Source: CAD feature listing. Evaluate the final solid. Frame: model axes, mm. A direction names the side the tool comes from. Coordinates: 2 decimals unless noted, no trailing zeros. Write each loop counter-clockwise with the first axis right and the second up, starting at its lowest first coordinate (ties: lowest second). Pieces come first, ordered by that corner, then holes. Notation, with made-up numbers: M -23,4 L 5,4 A10 cw 5,9 Z; hole C -31.5,48.25 d7. An arc over 180 degrees is marked long. Answer as CSV lines item,"result". Start each with the question number.
1. Line query: probe 1 along Y at (x, z) = (12, 187.17); probe 2 along Z at (x, y) = (-11, 0); probe 3 along Z at (x, y) = (0, 0). Output: solid intervals per line, ascending. Write a range as [from, to].
2. Mould query, pull axis Y, two halves, no side actions, for faces 4 (the face through (0.993, 2.628, 178.824)), 5 (the face through (26, 0, 145)), 6 (the face through (-2.17, -9.76, -39.44)). Classes: pulls with the +Y half, pulls with the -Y half, needs draft (parallel to the pull), parting line crosses it, or undercut.
3. Contact query for flat-ended pins moving along their axis: pin 1 Ø4.5 at (y, z) = (21.5, 159.5) entering from -X; pin 2 Ø10.5 at (y, z) = (0, 187.17) entering from -X; pin 3 Ø1.5 at (x, y) = (-12.5, 1.5) entering from -Z; pin 4 Ø4.5 at (x, z) = (-24, 96.5) entering from +Y. Output: stop coordinate, or through.
4. Section B-B on x = 0. Return the cut outline in (y, z), plus the area to 3 significant figures.
5. Section A-A on z = 187.17. Return the cut outline in (x, y) (3 decimals), plus the area to 3 significant figures.
6. Section C-C on z = 271. Return the cut outline in (x, y).
7. Reachability of faces 1 (the face through (-22, 20, 145)), 2 (the face through (22, 20, 145)), 3 (the face through (0, 27.5, 145)) from +Z, -Z, +X, -X, +Y, -Y: full face, straight path, thin tool, end or side. Return the list, or none.
8. Section D-D on y = 24. Return the cut outline in (x, z), plus the area to 3 significant figures.
```python
from build123d import *

# Parameters (mm, degrees)
BOSS_EXTRUDE1_DEPTH          = 295
SKETCH3_R                    = 10
BOSS_EXTRUDE3_DEPTH          = 80
M20_TAPPED_HOLE1_D           = 17.5
M20_TAPPED_HOLE1_CSINK_D     = 20.05
M20_TAPPED_HOLE1_CSINK_ANGLE = 90


with BuildPart() as part:
    # Sketch1 → Boss-Extrude1 (new body)
    with BuildSketch(Plane.XY):
        Polygon((-26, -12.5), (26, -12.5), (26, 12.5), (22, 12.5), (22, 27.5), (-22, 27.5), (-22, 12.5), (-26, 12.5), align=None)
    extrude(amount=BOSS_EXTRUDE1_DEPTH)

    # Sketch3 → Boss-Extrude3 (add)
    with BuildSketch(Plane.XY):
        Circle(SKETCH3_R)
    extrude(amount=-BOSS_EXTRUDE3_DEPTH)

    # M20 Tapped Hole1 (through all)
    with Locations(Plane.ZY.offset(26)):
        with Locations((187.17, 0)):
            CounterSinkHole(M20_TAPPED_HOLE1_D / 2, M20_TAPPED_HOLE1_CSINK_D / 2, counter_sink_angle=M20_TAPPED_HOLE1_CSINK_ANGLE)


solid = part.part
```
Values:
1,probe 1,"[-12.5, -8.75], [8.75, 27.5]"
1,probe 2,"[0, 178.42], [195.92, 295]"
1,probe 3,"[-80, 178.42], [195.92, 295]"
2,face 4,"undercut"
2,face 5,"needs draft"
2,face 6,"parting line crosses it"
3,pin 1,"x = -22"
3,pin 2,"through"
3,pin 3,"z = 0"
3,pin 4,"y = 27.5"
4,outline,"M -12.5,0 L -10,0 L -10,-80 L 10,-80 L 10,0 L 27.5,0 L 27.5,295 L -12.5,295 Z; hole C 0,187.17 d17.5"
4,area,"13,200 mm²"
5,outline,"M -26,-12.5 L 26,-12.5 L 26,-8.75 L -24.725,-8.75 L -26,-10.025 Z; M -26,10.025 L -24.725,8.75 L 26,8.75 L 26,12.5 L 22,12.5 L 22,27.5 L -22,27.5 L -22,12.5 L -26,12.5 Z"
5,area,"1,050 mm²"
6,outline,"M -26,-12.5 L 26,-12.5 L 26,12.5 L 22,12.5 L 22,27.5 L -22,27.5 L -22,12.5 L -26,12.5 Z"
7,face 1,"+Z, -Z, -X, +Y"
7,face 2,"+Z, -Z, +X, +Y"
7,face 3,"+Z, -Z, +X, -X, +Y"
8,outline,"M -22,0 L 22,0 L 22,295 L -22,295 Z"
8,area,"13,000 mm²"
